```python
from build123d import *

# Parameters (mm, degrees)
SKETCH3_W           = 38.1
SKETCH3_H           = 38.1
BOSS_EXTRUDE1_DEPTH = 48.26
SKETCH4_R           = 6.35
BOSS_EXTRUDE2_DEPTH = 38.1
SKETCH5_R           = 2.413
CUT_EXTRUDE1_DEPTH  = 10.16


with BuildPart() as part:
    # Sketch3 → Boss-Extrude1 (new body)
    with BuildSketch(Plane.XY):
        Rectangle(SKETCH3_W, SKETCH3_H)
    extrude(amount=-BOSS_EXTRUDE1_DEPTH)

    # Sketch4 → Boss-Extrude2 (add)
    with BuildSketch(Plane.XY):
        with Locations(Location((0, 0, 0), (0, 0, 180))):
            Circle(SKETCH4_R)
    extrude(amount=BOSS_EXTRUDE2_DEPTH)

    # Sketch5 → Cut-Extrude1 (cut)
    with BuildSketch(Plane(origin=(0, 19.05, 0), x_dir=(1, 0, 0), z_dir=(0, 1, 0))):
        with Locations(Location((-9.525, 44.45, 0), (0, 0, 270))):
            Circle(SKETCH5_R)
        with Locations(Location((9.525, 44.45, 0), (0, 0, 270))):
            Circle(SKETCH5_R)
        with Locations(Location((9.525, 7.62, 0), (0, 0, 270))):
            Circle(SKETCH5_R)
        with Locations(Location((-9.525, 7.62, 0), (0, 0, 270))):
            Circle(SKETCH5_R)
    extrude(amount=-CUT_EXTRUDE1_DEPTH, mode=Mode.SUBTRACT)


solid = part.part
```
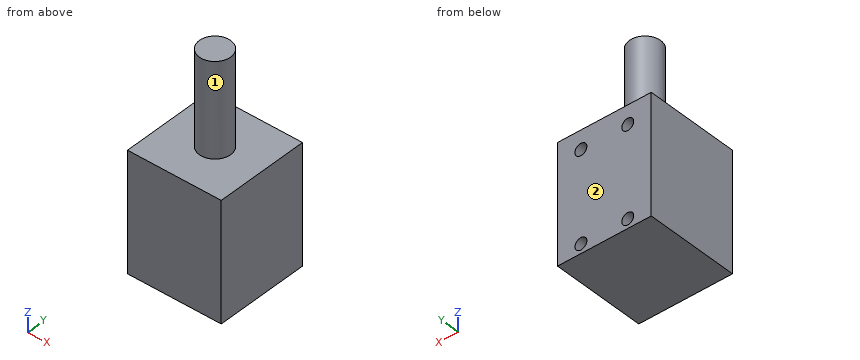
For this review, take the finished solid that the model builds, in its own axes (mm). Face numbers are marked on the shaded views. A direction names the side the tool comes from. Round coordinates to 2 decimals unless told otherwise and drop trailing zeros. Write each loop counter-clockwise with the first axis right and the second up, starting at its lowest first coordinate (ties: lowest second). Pieces come first, ordered by that corner, then holes.
1) For line 1 along X through (y, z) = (12, -44.45); line 2 along X through (y, z) = (12, -7); line 3 along Z through (x, y) = (-10.5, 3), list the stretches that pass through material, from the lowest coordinate up.
Answer below:
line 1: x = -19.05 to -11.94, -7.11 to 7.11, 11.94 to 19.05
line 2: x = -19.05 to -11.86, -7.19 to 7.19, 11.86 to 19.05
line 3: z = -48.26 to 0
2) Take a section at C-C on y = 10.5. Give the boundary of the cut face in (x, z) (3 decimals).
Answer below:
outline: (-19.05, -48.26) - (19.05, -48.26) - (19.05, 0) - (-19.05, 0) - close; hole circle Ø4.826 at (-9.525, -44.45); hole circle Ø4.826 at (-9.525, -7.62); hole circle Ø4.826 at (9.525, -44.45); hole circle Ø4.826 at (9.525, -7.62)
3) Machinability: for the marked faces 1 and 2, which of the approach directions +Z, -Z, +X, -X, +Y, -Y give a long, thin tool a straight path to every point of the face, cutting with its end or side? Answer none if there is none.
Answer below:
face 1: +Z
face 2: +Z, -Z, +X, -X, +Y
4) Take a section at A-A on y = 0. Give the boundary of the cut face in (x, z).
Answer below:
outline: (-19.05, -48.26) - (19.05, -48.26) - (19.05, 0) - (6.35, 0) - (6.35, 38.1) - (-6.35, 38.1) - (-6.35, 0) - (-19.05, 0) - close
5) Insertion check: pin 1 Ø5 at (x, y) = (-5.5, -11.5) entering from +Z; pin 2 Ø6 at (x, z) = (6.5, 24.5) entering from -Y; pin 3 Ø3 at (x, z) = (9.525, -7.62) entering from +Y. Each pin has a flat end and moves straight along its axis. Give the tip position at first contact, or say it passes through.
Answer below:
pin 1: stops at z = 0
pin 2: stops at y = -5.3
pin 3: stops at y = 8.89
6) Take a section at D-D on z = -44.45. Give the boundary of the cut face in (x, y).
Answer below:
outline: (-19.05, -19.05) - (19.05, -19.05) - (19.05, 19.05) - (11.94, 19.05) - (11.94, 8.89) - (7.11, 8.89) - (7.11, 19.05) - (-7.11, 19.05) - (-7.11, 8.89) - (-11.94, 8.89) - (-11.94, 19.05) - (-19.05, 19.05) - close
